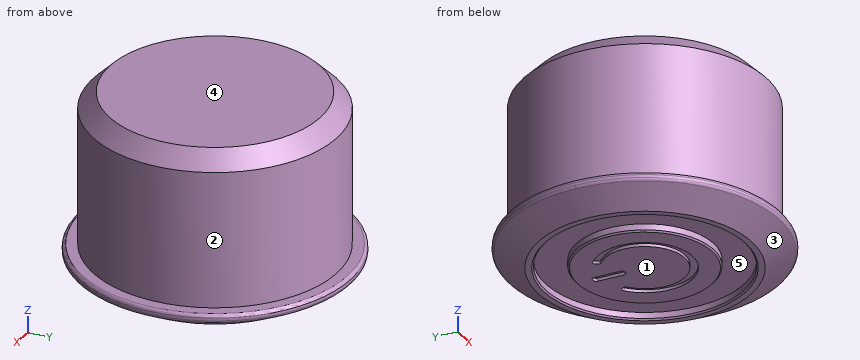
```python
from build123d import *

# Parameters (mm, degrees)
SKETCH_2_R          = 8.9
EXTRUDE_1_DEPTH     = 1.6
SKETCH_4_R          = 8
EXTRUDE_2_DEPTH     = 10
SKETCH_7_R          = 6.5
SKETCH_7_R_2        = 4.5
CUT_EXTRUDE_1_DEPTH = 0.5
CUT_EXTRUDE_2_DEPTH = 0.2
CHAMFER_1_SIZE      = 0.1
FILLET_1_R          = 0.2


# Read off the part's stored shape, not the designer's step: M16 机械螺纹 螺柱1
with BuildPart() as part:
    # 草图2 → 凸台-拉伸1 (new body)
    with BuildSketch(Plane.XY):
        Circle(SKETCH_2_R)
    extrude(amount=EXTRUDE_1_DEPTH)

    # 草图3 → 切除-旋转1 (revolve, cut)
    with BuildSketch(Plane(origin=(0, 0, 0), x_dir=(1, 0, 0), z_dir=(0, 1, 0))):
        Polygon((-8.9, -1.1), (-7, 0), (-8.9, 0), align=None)
    revolve(axis=Axis((0, 0, -2.565533084), (0, 0, 1)), mode=Mode.SUBTRACT)

    # 草图4 → 凸台-拉伸2 (add)
    with BuildSketch(Plane.XY.offset(1.6)):
        Circle(SKETCH_4_R)
    extrude(amount=EXTRUDE_2_DEPTH)

    # M16 机械螺纹 螺柱1 outline → M16 机械螺纹 螺柱1 (revolve, cut)
    with BuildSketch(Plane.XZ):
        Polygon((8, 11.6), (6.9175, 11.6), (8, 10.5175), align=None)
    revolve(axis=Axis((0, 0, 0), (0, 0, 1)), mode=Mode.SUBTRACT)

    # 草图7 → 切除-拉伸1 (cut)
    with BuildSketch(Plane(origin=(0, 0, 0), x_dir=(-1, 0, 0), z_dir=(0, 0, -1))):
        Circle(SKETCH_7_R)
        Circle(SKETCH_7_R_2, mode=Mode.SUBTRACT)
    extrude(amount=-CUT_EXTRUDE_1_DEPTH, mode=Mode.SUBTRACT)

    # 草图8 → 切除-拉伸2 (cut)
    with BuildSketch(Plane(origin=(0, 0, 0), x_dir=(-1, 0, 0), z_dir=(0, 0, -1))):
        with BuildLine():
            Line((1.643434087, 2.281182047), (1.702030214, 2.362516878))
            ThreePointArc((1.702030214, 2.362516878), (1.839011457, 2.444004167), (1.992055967, 2.399491052))
            ThreePointArc((1.992055967, 2.399491052), (0, -3.11862859), (-1.992055967, 2.399491052))
            ThreePointArc((-1.992055967, 2.399491052), (-1.839011457, 2.444004167), (-1.702030214, 2.362516878))
            Line((-1.702030214, 2.362516878), (-1.643434087, 2.281182047))
            ThreePointArc((-1.643434087, 2.281182047), (-1.607282835, 2.139224365), (-1.677581098, 2.010705686))
            ThreePointArc((-1.677581098, 2.010705686), (0, -2.61862859), (1.677581098, 2.010705686))
            ThreePointArc((1.677581098, 2.010705686), (1.607282835, 2.139224365), (1.643434087, 2.281182047))
        make_face()
        with BuildLine():
            Line((-0.050122003, 1.280793561), (0.050122003, 1.280793561))
            ThreePointArc((0.050122003, 1.280793561), (0.191543359, 1.339372204), (0.250122003, 1.480793561))
            Line((0.250122003, 1.480793561), (0.250122003, 3.214947097))
            ThreePointArc((0.250122003, 3.214947097), (0.191543359, 3.356368453), (0.050122003, 3.414947097))
            Line((0.050122003, 3.414947097), (-0.050122003, 3.414947097))
            ThreePointArc((-0.050122003, 3.414947097), (-0.191543359, 3.356368453), (-0.250122003, 3.214947097))
            Line((-0.250122003, 3.214947097), (-0.250122003, 1.480793561))
            ThreePointArc((-0.250122003, 1.480793561), (-0.191543359, 1.339372204), (-0.050122003, 1.280793561))
        make_face()
    extrude(amount=-CUT_EXTRUDE_2_DEPTH, mode=Mode.SUBTRACT)

    # 倒角1
    chamfer_1_edges = [part.edges().sort_by_distance(p)[0] for p in [
        (6.5, 0, 0),
        (4.5, 0, 0),
    ]]
    chamfer(chamfer_1_edges, length=CHAMFER_1_SIZE)

    # 圆角1
    fillet_1_edges = [part.edges().sort_by_distance(p)[0] for p in [
        (-8.9, 0, 1.6),
        (0, 8.9, 1.1),
    ]]
    fillet(fillet_1_edges, radius=FILLET_1_R)


solid = part.part
```
Design review of the part built by this model. Coordinates are the model's own, in mm. Face numbers are marked on the shaded views. A direction names the side the tool comes from. Round coordinates to 2 decimals unless told otherwise and drop trailing zeros. Write each loop counter-clockwise with the first axis right and the second up, starting at its lowest first coordinate (ties: lowest second). Pieces come first, ordered by that corner, then holes. Notation, with made-up numbers: (-28.75, 9) -> (-14.75, 9) arc R19 ccw to (-14.75, 37) -> close; hole circle Ø1 at (68.5, -40). An arc over 180 degrees is marked (long way). Answer in a Markdown table with one row per item.
Q1. To check wall thickness, follow L1, parallel to Y at x = 0, z = 0.25; L2, parallel to Y at x = 0, z = 0.4; L3, parallel to Z at x = -3, y = -4.5. State the ranges of each line that lie inside material, in increasing order. Write a range as [from, to].
The answers:
| item | result |
|---|---|
| L1 | [-7.43, -6.5], [-4.5, 4.5], [6.5, 7.43] |
| L2 | [-7.69, -6.5], [-4.5, 4.5], [6.5, 7.69] |
| L3 | [0.5, 11.6] |
Q2. Clearance check with flat-ended pins moving along their axes: pin 1 Ø5 at (y, z) = (5, 2) entering from -X; pin 2 Ø1 at (x, z) = (-3, 4.5) entering from -Y; pin 3 Ø1 at (x, z) = (0.5, 5) entering from +Y. State where each tip first meets the part, or that it passes through.
The answers:
| item | result |
|---|---|
| pin 1 | x = -8.52 |
| pin 2 | y = -7.6 |
| pin 3 | y = 8 |
Q3. For the marked faces 1 and 2, list the 3-axis set-ups (+Z, -Z, +X, -X, +Y, -Y) from which the entire face can be reached by the end or side of a thin tool; tool diameter is ignored.
The answers:
| item | result |
|---|---|
| face 1 | -Z, +X, -X, +Y, -Y |
| face 2 | +Z |
Q4. Draft analysis for pull direction X (two halves, no side actions). For the marked faces 3, 4 and 5, state which applies: +X half, -X half, draft (parallel to the pull), parting line (faces both ways), or undercut.
The answers:
| item | result |
|---|---|
| face 3 | parting line |
| face 4 | draft |
| face 5 | undercut |
Q5. Take a section at A-A, the plane z = 3. State the section outline as (x, y) points, then the cut area to 3 significant figures.
The answers:
| item | result |
|---|---|
| outline | circle Ø16 at (0, 0) |
| area | 201 mm² |
